Input: part model. Units: mm. Frame: model coordinates. A direction names the side the tool comes from. Coordinates: 2 decimals unless noted, no trailing zeros. Loops run counter-clockwise (first coordinate to the right, second up) from the corner with the lowest first, then second, coordinate; pieces in that order, holes last.
```python
from build123d import *

# Parameters (mm, degrees)
SKETCH1_R               = 8
BOSS_EXTRUDE1_DEPTH     = 20
SKETCH2_R               = 20
BOSS_EXTRUDE2_DEPTH     = 104
SKETCH3_R               = 15
CUT_EXTRUDE1_DEPTH      = 42
CUT_EXTRUDE1_DEPTH_BACK = 57
SKETCH4_W               = 4
SKETCH4_H               = 2.3
SKETCH5_R               = 4
CUT_EXTRUDE2_DEPTH      = 30
CIRPATTERN1_COUNT       = 6
FILLET1_R               = 3
CHAMFER1_SIZE           = 2


with BuildPart() as part:
    # Sketch1 → Boss-Extrude1 (new body)
    with BuildSketch(Plane.XY):
        with BuildLine():
            Line((41, -8), (41, -30))
            Line((41, -30), (-56, -30))
            Line((-56, -30), (-56, 40))
            Line((-56, 40), (41, 40))
            Line((41, 40), (41, 8))
            ThreePointArc((41, 8), (33, 0), (41, -8))
        make_face()
        with Locations((-41, 0)):
            Circle(SKETCH1_R, mode=Mode.SUBTRACT)
    extrude(amount=BOSS_EXTRUDE1_DEPTH)

    # Sketch2 → Boss-Extrude2 (add)
    with BuildSketch(Plane.XY.offset(20)):
        Circle(SKETCH2_R)
    extrude(amount=BOSS_EXTRUDE2_DEPTH)

    # Sketch3 → Cut-Extrude1 (cut, two sides)
    with BuildSketch(Plane(origin=(0, 0, 0), x_dir=(0, 0, -1), z_dir=(1, 0, 0))) as cut_extrude1_sk:
        with Locations((-90, 0)):
            Circle(SKETCH3_R)
    extrude(amount=CUT_EXTRUDE1_DEPTH, mode=Mode.SUBTRACT)
    extrude(cut_extrude1_sk.sketch, amount=-CUT_EXTRUDE1_DEPTH_BACK, mode=Mode.SUBTRACT)

    # Sketch4 → Cut-Revolve1 (revolve, cut)
    with BuildSketch(Plane(origin=(0, 0, 0), x_dir=(0, 0, -1), z_dir=(1, 0, 0))):
        with Locations((-72, 18.85)):
            Rectangle(SKETCH4_W, SKETCH4_H)
        with Locations((-64, 18.85)):
            Rectangle(SKETCH4_W, SKETCH4_H)
    revolve(axis=Axis((0, 0, 0), (0, 0, 1)), mode=Mode.SUBTRACT)

    # Sketch5 → Cut-Extrude2 (cut)
    with BuildSketch(Plane.XY.offset(124)):
        with Locations((10, 0)):
            Circle(SKETCH5_R)
    cut_extrude2 = extrude(amount=-CUT_EXTRUDE2_DEPTH, mode=Mode.SUBTRACT)

    # CirPattern1: Cut-Extrude2 ×6 about axis
    cirpattern1_axis = Axis((0, 0, 0), (0, 0, 1))
    for i in range(1, CIRPATTERN1_COUNT):
        add(cut_extrude2.rotate(cirpattern1_axis, i * 360 / CIRPATTERN1_COUNT), mode=Mode.SUBTRACT)

    # Fillet1
    fillet1_edges = [part.edges().sort_by_distance(p)[0] for p in [
        (-56, -30, 10),
        (-56, 40, 10),
    ]]
    fillet(fillet1_edges, radius=FILLET1_R)

    # Chamfer1
    chamfer1_edges = [part.edges().sort_by_distance(p)[0] for p in [
        (-20, 0, 124),
    ]]
    chamfer(chamfer1_edges, length=CHAMFER1_SIZE)


solid = part.part
```
Item 1: Section query D-D (y = 31). Output: boundary loops of the cut face in (x, z), then the cut area to 3 significant figures.
Result:
outline: (-56, 0) - (41, 0) - (41, 20) - (-56, 20) - close
area: 1,940 mm2
Item 2: Reachability of faces 5 (the face through (-5.867, -12.565, 114.088)), 6 (the face through (-55.1, -29.14, 10.14)), 7 (the face through (-5.32, 16.88, 63.97)) from +Z, -Z, +X, -X, +Y, -Y: full face, straight path, thin tool, end or side. Return the list, or none.
Result:
face 5: +Z
face 6: +Z, -Z, -X, -Y
face 7: none
Item 3: Section query A-A (z = 15). Output: boundary loops of the cut face in (x, y), then the cut area to 3 significant figures.
Result:
outline: (-56, -27) arc R3 ccw to (-53, -30) - (41, -30) - (41, -8) arc R8 cw to (41, 8) - (41, 40) - (-53, 40) arc R3 ccw to (-56, 37) - close; hole circle Ø16 at (-41, 0)
area: 6,480 mm2
Item 4: Contact query for flat-ended pins moving along their axis: P1, Ø20, axis at x = -2, y = 8, coming from the +Z side; P2, Ø8, axis at y = -9, z = 60.5, coming from the -X side; P3, Ø1, axis at y = 1.5, z = 25, coming from the +X side (3 decimals); P4, Ø6.5, axis at x = -5, y = 8.66, coming from the +Z side. Output: stop coordinate, or through.
Result:
P1: stops at z = 124
P2: stops at x = -19.36
P3: stops at x = 19.975
P4: stops at z = 80.88
Item 5: Section query C-C (z = 111). Output: boundary loops of the cut face in (x, y).
Result:
outline: circle Ø40 at (0, 0); hole circle Ø8 at (-10, 0); hole circle Ø8 at (-5, -8.66); hole circle Ø8 at (-5, 8.66); hole circle Ø8 at (5, -8.66); hole circle Ø8 at (5, 8.66); hole circle Ø8 at (10, 0)
Item 6: Section query B-B (x = -41). Output: boundary loops of the cut face in (y, z).
Result:
outline: (-30, 0) - (-8, 0) - (-8, 20) - (-30, 20) - close; (8, 0) - (40, 0) - (40, 20) - (8, 20) - close
Item 7: Line query: L1, parallel to Y at x = -41, z = 6; L2, parallel to Y at x = 5, z = 113; L3, parallel to Z at x = -13.5, y = -15.5. Output: solid intervals per line, ascending.
Result:
L1: y = -30 to -8, 8 to 40
L2: y = -19.36 to -12.66, -4.66 to 4.66, 12.66 to 19.36
L3: z = 0 to 20
Item 8: Mould query, pull axis X, two halves, no side actions, for faces 1 (the face through (5.867, 12.565, 114.088)), 2 (the face through (6, 0, 114)), 3 (the face through (-18, 13, 20)), 4 (the face through (-55.14, 39.1, 10.14)). Classes: +X half, -X half, draft (parallel to the pull), parting line (faces both ways), or undercut.
Result:
face 1: undercut
face 2: undercut
face 3: draft
face 4: -X half
